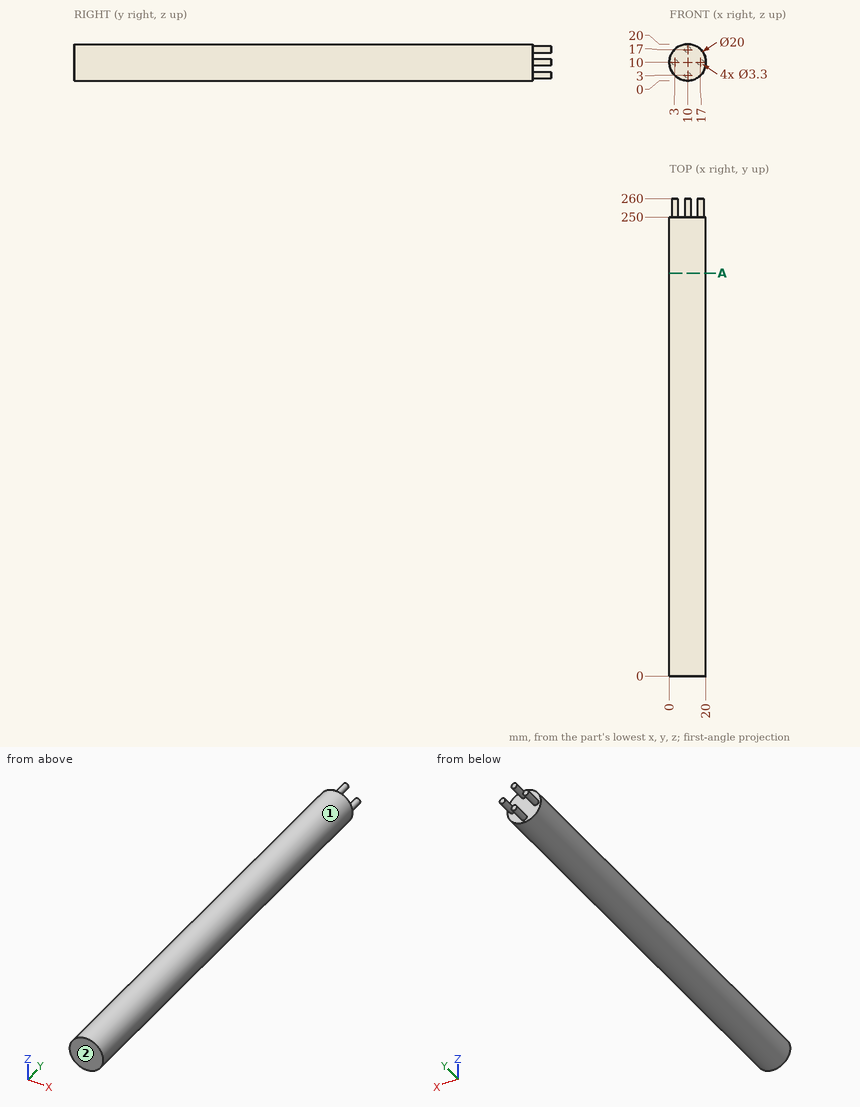
Part print with two shaded views. Sizes in mm from the minimum x, y, z corner. Give positions to 0.01 mm unless a question says otherwise; leave off trailing zeros. Order: outer loops, then holes, each group sorted by start corner. A loop starts at its lowest first (then second) coordinate and runs counter-clockwise, first axis right, second up.
(1) Drill centre lines: L1, parallel to Y at x = 11, z = 19.25; L2, parallel to Z at x = 9.75, y = 171; L3, parallel to Z at x = 15.25, y = 154. Where is each one in solid material? Low to high.
(2) Saw through at A-A, the plane y = 219.5. Give the cut face in (x, z), then the cut area to 3 significant figures.
(3) Mould opens along Z. For the marked faces 1 and 2 say: released by +Z, released by -Z, zero draft, split by the parting line, or undercut.
(4) Flat gauge pins, fed straight in: pin 1 (3 mm diameter, centred on y = 77.5, z = 6, fed in from +X); pin 2 (1 mm diameter, centred on x = 6.5, z = 16.5, fed in from +Y); pin 3 (12 mm diameter, centred on x = 3.5, y = 80.5, fed in from +Z). Where does each tip first touch, or does it go through?
Results found:
1. L1: y = 0 to 250
1. L2: z = 0 to 20
1. L3: z = 1.49 to 18.51
2. outline: circle Ø20 at (10, 10)
2. area: 314 mm2
3. face 1: split by the parting line
3. face 2: zero draft
4. pin 1: stops at x = 19.68
4. pin 2: stops at y = 250
4. pin 3: stops at z = 19.99
